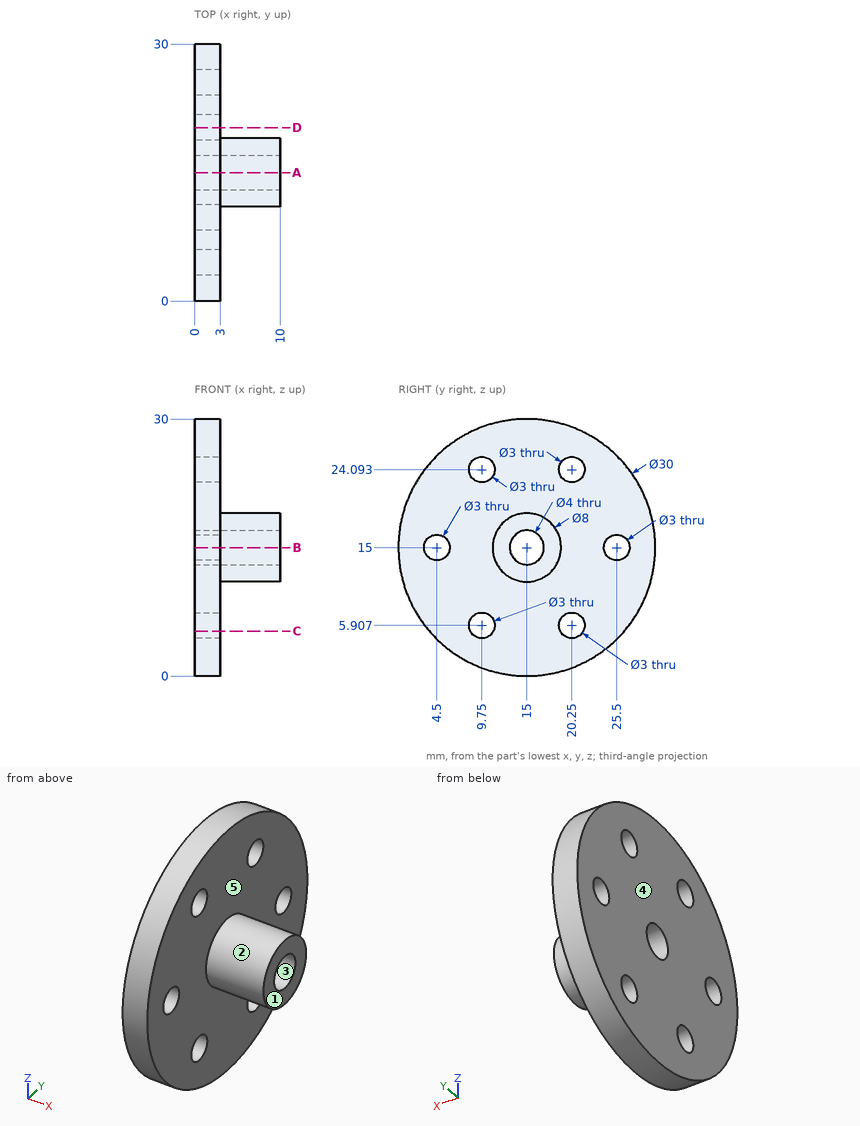
Check sheet for the drawn part. Datum: minimum x, y, z corner. Units: mm. A direction names the side the tool comes from. Give positions to 0.01 mm unless a question says otherwise; leave off trailing zeros. Loops run counter-clockwise (first coordinate to the right, second up) from the corner with the lowest first, then second, coordinate; pieces in that order, holes last.
1) Thickness scan on line 1 along Y through (x, z) = (7.75, 15); line 2 along Y through (x, z) = (2.05, 15). Record the ranges inside material, lowest first.
2) Sectioned sample at A-A, the plane y = 15. Enter the section's corners in (x, z).
3) Depth check by flat-ended pin: pin 1 Ø4 at (y, z) = (20.25, 5.91) entering from -X; pin 2 Ø4 at (y, z) = (5.5, 15.5) entering from +X; pin 3 Ø5 at (x, y) = (3, 19) entering from -Z (1 decimal); pin 4 Ø1 at (x, z) = (8.5, 17.5) entering from +Y. Enter the tip coordinate at first touch or a pass-through.
4) Draft check along Y on the marked faces 1, 2 and 3. Enter one of: pulls with the +Y half, pulls with the -Y half, needs draft (parallel to the pull), parting line crosses it, or undercut.
5) Sectioned sample at B-B, the plane z = 15. Enter the section's corners in (x, y), then the cut area to 3 significant figures.
6) Set-up check for the marked faces 4 and 5: record each of +Z, -Z, +X, -X, +Y, -Y from which the full face is reachable in a straight line by a thin tool's end or side.
7) Sectioned sample at D-D, the plane y = 20.25. Enter the section's corners in (x, z).
8) Sectioned sample at C-C, the plane z = 5.25. Enter the section's corners in (x, y).
Answers:
1. line 1: y = 11 to 13, 17 to 19
1. line 2: y = 0 to 3, 6 to 13, 17 to 24, 27 to 30
2. outline: (0, 0) - (3, 0) - (3, 11) - (10, 11) - (10, 13) - (0, 13) - close; (0, 17) - (10, 17) - (10, 19) - (3, 19) - (3, 30) - (0, 30) - close
3. pin 1: stops at x = 0
3. pin 2: stops at x = 3
3. pin 3: stops at z = 0.1
3. pin 4: stops at y = 18.46
4. face 1: needs draft
4. face 2: parting line crosses it
4. face 3: undercut
5. outline: (0, 0) - (3, 0) - (3, 3) - (0, 3) - close; (0, 6) - (3, 6) - (3, 11) - (10, 11) - (10, 13) - (0, 13) - close; (0, 17) - (10, 17) - (10, 19) - (3, 19) - (3, 24) - (0, 24) - close; (0, 27) - (3, 27) - (3, 30) - (0, 30) - close
5. area: 88.0 mm2
6. face 4: +Z, -Z, -X, +Y, -Y
6. face 5: +X
7. outline: (0, 0.95) - (3, 0.95) - (3, 4.41) - (0, 4.41) - close; (0, 7.41) - (3, 7.41) - (3, 22.59) - (0, 22.59) - close; (0, 25.59) - (3, 25.59) - (3, 29.05) - (0, 29.05) - close
8. outline: (0, 3.6) - (3, 3.6) - (3, 8.4) - (0, 8.4) - close; (0, 11.1) - (3, 11.1) - (3, 18.9) - (0, 18.9) - close; (0, 21.6) - (3, 21.6) - (3, 26.4) - (0, 26.4) - close
